Model file for the job. Use its own axes, mm. A direction names the side the tool comes from. Round coordinates to 2 decimals unless told otherwise and drop trailing zeros. Order: outer loops, then holes, each group sorted by start corner. A loop starts at its lowest first (then second) coordinate and runs counter-clockwise, first axis right, second up. Notation, with made-up numbers: M 13.25,-33 L 54.25,-33 A24 ccw 54.25,-10 Z; hole C -26.5,-4 d4. An arc over 180 degrees is marked long. Return JSON: item names as keys, results as strings. Group by question number.
Item 1: Slice it at B-B on y = -33.5. Write the cut outline in (x, z), then the cut area to 3 significant figures.
Item 2: Pull direction Y, two halves, no side cores. Call faces 5 (the face through (-27.418, -22.274, 12.325)), 6 (the face through (-44.434, 32.413, 12.325)), 7 (the face through (31.873, -37.308, 12.325)): pulls with the +Y half, pulls with the -Y half, needs draft (parallel to the pull), parting line crosses it, or undercut.
Item 3: Slice it at C-C on y = -18. Write the cut outline in (x, z), then the cut area to 3 significant figures.
Item 4: Pin check, flat tips, straight feed: pin 1 Ø3 at (y, z) = (14.5, 13.5) entering from -X; pin 2 Ø1.1 at (x, z) = (-0.5, 18) entering from -Y; pin 3 Ø3 at (y, z) = (40, 17) entering from -X; pin 4 Ø9 at (x, y) = (25.78, 14.88) entering from +Z. Stop position of each tip, or through.
Item 5: Which spindle directions (+Z, -Z, +X, -X, +Y, -Y) get a long thin tool onto all of the face, cutting with end or side? Do faces 1 (the face through (-55, 0, 12)), 2 (the face through (47.715, -11.449, 12.325)), 3 (the face through (3.86, -48.92, 12.32)), 4 (the face through (3.9, 49, 12.3)). Say none if no direction does.
Item 6: Slice it at A-A on x = 31. Write the cut outline in (y, z).
Item 7: Probe line 1 along X through (y, z) = (0.5, 7); line 2 along Y through (x, z) = (-19, 11.5); line 3 along Y through (x, z) = (24, 17.25). List the from-to ranges inside material, lowest first.
Item 8: Slice it at D-D on z = 12. Give the number of separate pieces and of enclosed holes in the cut face, then the cut area to 3 significant figures.
from build123d import *

# Parameters (mm, degrees)
F0_R     = 7.572247
F0_R_2   = 1.775
F0_R_3   = 4
F1_DEPTH = 25


with BuildPart() as f1:
    # F0 (on Top) → F1 (new body)
    with BuildSketch(Plane.XY):
        with BuildLine():
            ThreePointArc((-5.309504, 51.742404), (-7.086811, 53.712393), (-9.705882, 54.136825))
            ThreePointArc((-9.705882, 54.136825), (-16.995935, 52.308108), (-23.968604, 49.502586))
            ThreePointArc((-23.968604, 49.502586), (-25.838002, 47.619762), (-26.117943, 44.981332))
            Line((-26.117943, 44.981332), (-25.161306, 38.789124))
            ThreePointArc((-25.161306, 38.789124), (-25.291556, 37.714888), (-25.962287, 36.865731))
            Line((-25.962287, 36.865731), (-27.038606, 36.083739))
            ThreePointArc((-27.038606, 36.083739), (-28.053469, 35.708241), (-29.115378, 35.916322))
            Line((-29.115378, 35.916322), (-34.708901, 38.739636))
            ThreePointArc((-34.708901, 38.739636), (-37.304703, 39.288716), (-39.673051, 38.092637))
            ThreePointArc((-39.673051, 38.092637), (-44.495935, 32.328189), (-48.487898, 25.960042))
            ThreePointArc((-48.487898, 25.960042), (-48.893577, 23.338), (-47.569223, 21.03892))
            Line((-47.569223, 21.03892), (-43.155599, 16.591616))
            ThreePointArc((-43.155599, 16.591616), (-42.629554, 15.645982), (-42.673064, 14.564754))
            Line((-42.673064, 14.564754), (-43.084182, 13.299464))
            ThreePointArc((-43.084182, 13.299464), (-43.684511, 12.399158), (-44.66592, 11.943325))
            Line((-44.66592, 11.943325), (-50.850677, 10.939644))
            ThreePointArc((-50.850677, 10.939644), (-53.273467, 9.858085), (-54.486463, 7.498356))
            ThreePointArc((-54.486463, 7.498356), (-55, 0), (-54.486463, -7.498356))
            ThreePointArc((-54.486463, -7.498356), (-53.273467, -9.858085), (-50.850677, -10.939644))
            Line((-50.850677, -10.939644), (-44.66592, -11.943325))
            ThreePointArc((-44.66592, -11.943325), (-43.684511, -12.399158), (-43.084182, -13.299464))
            Line((-43.084182, -13.299464), (-42.673064, -14.564754))
            ThreePointArc((-42.673064, -14.564754), (-42.629554, -15.645982), (-43.155599, -16.591616))
            Line((-43.155599, -16.591616), (-47.569223, -21.03892))
            ThreePointArc((-47.569223, -21.03892), (-48.893577, -23.338), (-48.487898, -25.960042))
            ThreePointArc((-48.487898, -25.960042), (-44.495935, -32.328189), (-39.673051, -38.092637))
            ThreePointArc((-39.673051, -38.092637), (-37.304703, -39.288716), (-34.708901, -38.739636))
            Line((-34.708901, -38.739636), (-29.115378, -35.916322))
            ThreePointArc((-29.115378, -35.916322), (-28.053469, -35.708241), (-27.038606, -36.083739))
            Line((-27.038606, -36.083739), (-25.962287, -36.865731))
            ThreePointArc((-25.962287, -36.865731), (-25.291556, -37.714888), (-25.161306, -38.789124))
            Line((-25.161306, -38.789124), (-26.117943, -44.981332))
            ThreePointArc((-26.117943, -44.981332), (-25.838002, -47.619762), (-23.968604, -49.502586))
            ThreePointArc((-23.968604, -49.502586), (-16.995935, -52.308108), (-9.705882, -54.136825))
            ThreePointArc((-9.705882, -54.136825), (-7.086811, -53.712393), (-5.309504, -51.742404))
            Line((-5.309504, -51.742404), (-2.443751, -46.170505))
            ThreePointArc((-2.443751, -46.170505), (-1.706956, -45.377989), (-0.665202, -45.085252))
            Line((-0.665202, -45.085252), (0.665202, -45.085252))
            ThreePointArc((0.665202, -45.085252), (1.706956, -45.377989), (2.443751, -46.170505))
            Line((2.443751, -46.170505), (5.309504, -51.742404))
            ThreePointArc((5.309504, -51.742404), (7.086811, -53.712393), (9.705882, -54.136825))
            ThreePointArc((9.705882, -54.136825), (16.995935, -52.308108), (23.968604, -49.502586))
            ThreePointArc((23.968604, -49.502586), (25.838002, -47.619762), (26.117943, -44.981332))
            Line((26.117943, -44.981332), (25.161306, -38.789124))
            ThreePointArc((25.161306, -38.789124), (25.291556, -37.714888), (25.962287, -36.865731))
            Line((25.962287, -36.865731), (27.038606, -36.083739))
            ThreePointArc((27.038606, -36.083739), (28.053469, -35.708241), (29.115378, -35.916322))
            Line((29.115378, -35.916322), (34.708901, -38.739636))
            ThreePointArc((34.708901, -38.739636), (37.304703, -39.288716), (39.673051, -38.092637))
            ThreePointArc((39.673051, -38.092637), (44.495935, -32.328189), (48.487898, -25.960042))
            ThreePointArc((48.487898, -25.960042), (48.893577, -23.338), (47.569223, -21.03892))
            Line((47.569223, -21.03892), (43.155599, -16.591616))
            ThreePointArc((43.155599, -16.591616), (42.629554, -15.645982), (42.673064, -14.564754))
            Line((42.673064, -14.564754), (43.084182, -13.299464))
            ThreePointArc((43.084182, -13.299464), (43.684511, -12.399158), (44.66592, -11.943325))
            Line((44.66592, -11.943325), (50.850677, -10.939644))
            ThreePointArc((50.850677, -10.939644), (53.273467, -9.858085), (54.486463, -7.498356))
            ThreePointArc((54.486463, -7.498356), (55, 0), (54.486463, 7.498356))
            ThreePointArc((54.486463, 7.498356), (53.273467, 9.858085), (50.850677, 10.939644))
            Line((50.850677, 10.939644), (44.66592, 11.943325))
            ThreePointArc((44.66592, 11.943325), (43.684511, 12.399158), (43.084182, 13.299464))
            Line((43.084182, 13.299464), (42.673064, 14.564754))
            ThreePointArc((42.673064, 14.564754), (42.629554, 15.645982), (43.155599, 16.591616))
            Line((43.155599, 16.591616), (47.569223, 21.03892))
            ThreePointArc((47.569223, 21.03892), (48.893577, 23.338), (48.487898, 25.960042))
            ThreePointArc((48.487898, 25.960042), (44.495935, 32.328189), (39.673051, 38.092637))
            ThreePointArc((39.673051, 38.092637), (37.304703, 39.288716), (34.708901, 38.739636))
            Line((34.708901, 38.739636), (29.115378, 35.916322))
            ThreePointArc((29.115378, 35.916322), (28.053469, 35.708241), (27.038606, 36.083739))
            Line((27.038606, 36.083739), (25.962287, 36.865731))
            ThreePointArc((25.962287, 36.865731), (25.291556, 37.714888), (25.161306, 38.789124))
            Line((25.161306, 38.789124), (26.117943, 44.981332))
            ThreePointArc((26.117943, 44.981332), (25.838002, 47.619762), (23.968604, 49.502586))
            ThreePointArc((23.968604, 49.502586), (16.995935, 52.308108), (9.705882, 54.136825))
            ThreePointArc((9.705882, 54.136825), (7.086811, 53.712393), (5.309504, 51.742404))
            Line((5.309504, 51.742404), (2.443751, 46.170505))
            ThreePointArc((2.443751, 46.170505), (1.706956, 45.377989), (0.665202, 45.085252))
            Line((0.665202, 45.085252), (-0.665202, 45.085252))
            ThreePointArc((-0.665202, 45.085252), (-1.706956, 45.377989), (-2.443751, 46.170505))
            Line((-2.443751, 46.170505), (-5.309504, 51.742404))
        make_face()
        with Locations((-25.776053, -14.881811)):
            Circle(F0_R, mode=Mode.SUBTRACT)
        with Locations((-7.996251, -0.088927)):
            Circle(F0_R_2, mode=Mode.SUBTRACT)
        with Locations((0, -29.763622)):
            Circle(F0_R, mode=Mode.SUBTRACT)
        with Locations((25.776053, -14.881811)):
            Circle(F0_R, mode=Mode.SUBTRACT)
        with Locations((0.053749, -8.138927)):
            Circle(F0_R_2, mode=Mode.SUBTRACT)
        with Locations((0.053749, -0.088927)):
            Circle(F0_R_3, mode=Mode.SUBTRACT)
        with Locations((8.103749, -0.088927)):
            Circle(F0_R_2, mode=Mode.SUBTRACT)
        with Locations((-25.776053, 14.881811)):
            Circle(F0_R, mode=Mode.SUBTRACT)
        with Locations((0.053749, 7.961073)):
            Circle(F0_R_2, mode=Mode.SUBTRACT)
        with Locations((25.776053, 14.881811)):
            Circle(F0_R, mode=Mode.SUBTRACT)
        with Locations((0, 29.763622)):
            Circle(F0_R, mode=Mode.SUBTRACT)
    extrude(amount=F1_DEPTH)


solid = f1.part
Output values:
{
 "1": {"outline": "M -43.62,0 L -6.59,0 L -6.59,25 L -43.62,25 Z; M 6.59,0 L 43.62,0 L 43.62,25 L 6.59,25 Z", "area": "1,850 mm²"},
 "2": {"face 5": "undercut", "face 6": "pulls with the +Y half", "face 7": "pulls with the -Y half"},
 "3": {"outline": "M -44.55,0 L -32.68,0 L -32.68,25 L -44.55,25 Z; M -18.88,0 L 18.88,0 L 18.88,25 L -18.88,25 Z; M 32.68,0 L 44.55,0 L 44.55,25 L 32.68,25 Z", "area": "1,540 mm²"},
 "4": {"pin 1": "x = -43.21", "pin 2": "y = -45.12", "pin 3": "x = -39.22", "pin 4": "through"},
 "5": {"face 1": "+Z, -Z, -X", "face 2": "+Z, -Z, +X", "face 3": "+Z, -Z, -Y", "face 4": "+Z, -Z, +Y"},
 "6": {"outline": "M -36.87,0 L -20.36,0 L -20.36,25 L -36.87,25 Z; M -9.4,0 L 9.4,0 L 9.4,25 L -9.4,25 Z; M 20.36,0 L 36.87,0 L 36.87,25 L 20.36,25 Z"},
 "7": {"line 1": "-55 to -9.67, -6.32 to -3.9, 4.01 to 6.43, 9.78 to 55", "line 2": "-51.61 to -18.26, -11.5 to 11.5, 18.26 to 51.61", "line 3": "-49.49 to -22.24, -7.52 to 7.52, 22.24 to 49.49"},
 "8": {"separate pieces": "1", "enclosed holes": "11", "area": "7,450 mm²"}
}
